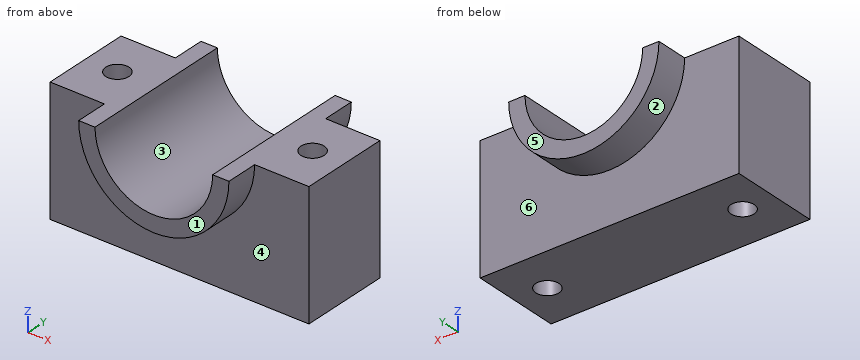
```python
from build123d import *

# Parameters (mm, degrees)
F1_DEPTH = 50.8
F2_DEPTH = 29.464
F5_D     = 15.24
F6_D     = 15.24


with BuildPart() as f1:
    # F0 (on Front) → F1 (new body, symmetric)
    with BuildSketch(Plane.XZ):
        with BuildLine():
            ThreePointArc((-49.268454, 41.154392), (0, -7.871612), (49.268454, 41.154392))
            Line((49.268454, 41.154392), (38.600289, 41.154392))
            ThreePointArc((38.600289, 41.154392), (0, 2.796388), (-38.600289, 41.154392))
            Line((-38.600289, 41.154392), (-49.268454, 41.154392))
        make_face()
    extrude(amount=F1_DEPTH, both=True)

    # F0 (on Front) → F2 (join, symmetric)
    with BuildSketch(Plane.XZ):
        with BuildLine():
            Line((-84.846668, -41.154392), (84.846668, -41.154392))
            Line((84.846668, -41.154392), (84.846668, 41.154392))
            Line((84.846668, 41.154392), (49.268454, 41.154392))
            ThreePointArc((49.268454, 41.154392), (0, -7.871612), (-49.268454, 41.154392))
            Line((-49.268454, 41.154392), (-84.846668, 41.154392))
            Line((-84.846668, 41.154392), (-84.846668, -41.154392))
        make_face()
        with BuildLine():
            ThreePointArc((-49.268454, 41.154392), (0, -7.871612), (49.268454, 41.154392))
            Line((49.268454, 41.154392), (38.600289, 41.154392))
            ThreePointArc((38.600289, 41.154392), (0, 2.796388), (-38.600289, 41.154392))
            Line((-38.600289, 41.154392), (-49.268454, 41.154392))
        make_face()
    extrude(amount=F2_DEPTH, both=True)

    # F5 (through all)
    with Locations(Plane.XY.offset(41.154392)):
        with Locations((-64.000289, 0)):
            Hole(F5_D / 2)

    # F6 (through all)
    with Locations(Plane.XY.offset(41.154392)):
        with Locations((64.000289, 0)):
            Hole(F6_D / 2)


solid = f1.part
```
Model file for the job. Use its own axes, mm. Face numbers are marked on the shaded views. A direction names the side the tool comes from. Coordinates: 2 decimals unless noted, no trailing zeros. Loops run counter-clockwise (first coordinate to the right, second up) from the corner with the lowest first, then second, coordinate; pieces in that order, holes last. Notation, with made-up numbers: (-7.5, -28.75) - (-2.5, -28.75) arc R29 ccw to (-2.5, 3.25) - close; hole circle Ø6 at (-39.5, -34.75). An arc over 180 degrees is marked (long way). Answer as a JSON object with one key per item and string values. Group by question number.
(1) Probe line 1 along X through (y, z) = (-3, 8); line 2 along Y through (x, z) = (-12, -31); line 3 along Y through (x, z) = (65.5, -21). List the from-to ranges inside material, lowest first.
(2) Flat gauge pins, fed straight in: pin 1 (24.5 mm diameter, centred on x = 34, z = -19.5, fed in from +Y); pin 2 (6 mm diameter, centred on x = 5, y = -3, fed in from +Z); pin 3 (12 mm diameter, centred on x = 64, y = 0, fed in from -Z); pin 4 (5 mm diameter, centred on x = 20.5, y = 25, fed in from +Z). Where does each tip first touch, or does it go through?
(3) Cut at D-D (z = -24.5). Give the cut face in (x, y), then the cut area to 3 significant figures.
(4) Two-plate mould, pull along X, no slides. Class the marked faces 1, 2 and 3: released by +X, released by -X, zero draft, split by the parting line, or undercut.
(5) Cut at A-A (y = 0). Give the cut face in (x, z).
(6) Cut at C-C (z = 10.5). Give the cut face in (x, y).
(7) Cut at B-B (x = -64). Give the cut face in (y, z).
(8) Tool access for the marked faces 4, 5 and 6: list every direction of +Z, -Z, +X, -X, +Y, -Y with a clear straight run to the whole face (end or side of a thin tool).
Geometry says:
{
 "1": {"line 1": "x = -84.85 to -71, -57 to -19.36, 19.36 to 57, 71 to 84.85", "line 2": "y = -29.46 to 29.46", "line 3": "y = -29.46 to -7.47, 7.47 to 29.46"},
 "2": {"pin 1": "stops at y = 29.46", "pin 2": "stops at z = 3.63", "pin 3": "passes through", "pin 4": "stops at z = 10.4"},
 "3": {"outline": "(-84.85, -29.46) - (84.85, -29.46) - (84.85, 29.46) - (-84.85, 29.46) - close; hole circle Ø15.24 at (-64, 0); hole circle Ø15.24 at (64, 0)", "area": "9,630 mm^2"},
 "4": {"face 1": "zero draft", "face 2": "split by the parting line", "face 3": "undercut"},
 "5": {"outline": "(-84.85, -41.15) - (-71.62, -41.15) - (-71.62, 41.15) - (-84.85, 41.15) - close; (-56.38, -41.15) - (56.38, -41.15) - (56.38, 41.15) - (38.6, 41.15) arc R38.6 cw to (-38.6, 41.15) - (-56.38, 41.15) - close; (71.62, -41.15) - (84.85, -41.15) - (84.85, 41.15) - (71.62, 41.15) - close"},
 "6": {"outline": "(-84.85, -29.46) - (-38.38, -29.46) - (-38.38, -50.8) - (-23.14, -50.8) - (-23.14, 50.8) - (-38.38, 50.8) - (-38.38, 29.46) - (-84.85, 29.46) - close; (23.14, -50.8) - (38.38, -50.8) - (38.38, -29.46) - (84.85, -29.46) - (84.85, 29.46) - (38.38, 29.46) - (38.38, 50.8) - (23.14, 50.8) - close; hole circle Ø15.24 at (-64, 0); hole circle Ø15.24 at (64, 0)"},
 "7": {"outline": "(-29.46, -41.15) - (-7.62, -41.15) - (-7.62, 41.15) - (-29.46, 41.15) - close; (7.62, -41.15) - (29.46, -41.15) - (29.46, 41.15) - (7.62, 41.15) - close"},
 "8": {"face 4": "-Z, -Y", "face 5": "+Z, -Z, +X, -X, +Y", "face 6": "-Z, +Y"}
}
